Here's how the part is built. I have some questions about the finished solid (model axes, mm). A direction names the side the tool comes from. Round coordinates to 2 decimals unless told otherwise and drop trailing zeros. Loops run counter-clockwise (first coordinate to the right, second up) from the corner with the lowest first, then second, coordinate; pieces in that order, holes last. Notation, with made-up numbers: M 60,74.5 L 72,74.5 A18 cw 72,83.5 Z; hole C -6.5,-9.75 d8. An arc over 180 degrees is marked long. Write each question's results on one line, items separated by ' | '. Start each with the question number.
```python
from build123d import *

# Parameters (mm, degrees)
SKETCH2_R           = 4.75
SKETCH2_R_2         = 3.75
BOSS_EXTRUDE1_DEPTH = 3.44
SKETCH3_W           = 4
SKETCH3_H           = 11.757601451
BOSS_EXTRUDE2_DEPTH = 1
SKETCH4_W           = 1.4
SKETCH4_H           = 4.6
CUT_EXTRUDE1_DEPTH  = 1
FILLET1_R           = 13
CHAMFER1_SIZE       = 0.5
FILLET2_R           = 1


with BuildPart() as part:
    # Sketch2 → Boss-Extrude1 (new body)
    with BuildSketch(Plane(origin=(0, 0, 0), x_dir=(1, 0, 0), z_dir=(0, 1, 0))):
        with Locations(Location((0, 0, 0), (0, 0, 270))):
            Circle(SKETCH2_R)
        with Locations(Location((0, 0, 0), (0, 0, 270))):
            Circle(SKETCH2_R_2, mode=Mode.SUBTRACT)
    extrude(amount=BOSS_EXTRUDE1_DEPTH)

    # Sketch3 → Boss-Extrude2 (add)
    with BuildSketch(Plane(origin=(-4.8, 0, 0), x_dir=(0, 0, -1), z_dir=(1, 0, 0))):
        with Locations((0, 5.878800726)):
            Rectangle(SKETCH3_W, SKETCH3_H)
    extrude(amount=BOSS_EXTRUDE2_DEPTH)

    # Sketch4 → Cut-Extrude1 (cut)
    with BuildSketch(Plane.ZY.offset(4.8)):
        with Locations((0, 8.46916965)):
            Rectangle(SKETCH4_W, SKETCH4_H)
    extrude(amount=-CUT_EXTRUDE1_DEPTH, mode=Mode.SUBTRACT)

    # Fillet1
    # the kernel refuses this fillet: 13 mm, written as the material it adds along each edge
    with BuildSketch(Plane(origin=(-4.308421985, 3.44, 2), x_dir=(0.5581025465687688, 0, 0.8297719852546573), z_dir=(0, -1, 0))) as fillet1_piece_1:
        with BuildLine():
            CenterArc((3.528934631, 12.839109145), FILLET1_R, 252.988692503, 7.987692365)
            Line((-0.274350942, 0.407897665), (-0.350416654, 0.159273436))
            ThreePointArc((-0.350416654, 0.159273436), (-0.352916187, 0.058842171), (-0.215740716, -0.145106662))
            Line((-0.215740716, -0.145106662), (0.0407788, -0.256782183))
            ThreePointArc((0.0407788, -0.256782183), (0.744997311, -0.201212957), (1.449215822, -0.256782183))
            Line((1.449215822, -0.256782183), (1.489994622, 0))
        make_face()
    extrude(amount=3.44)
    with BuildSketch(Plane(origin=(-4.308421985, 3.44, -2), x_dir=(0.5581025465687675, 0, -0.8297719852546583), z_dir=(0, -1, 0))) as fillet1_piece_2:
        with BuildLine():
            CenterArc((3.528934631, -12.839109145), FILLET1_R, 99.023615132, 7.987692365)
            Line((-0.274350942, -0.407897665), (-0.350416654, -0.159273436))
            ThreePointArc((-0.350416654, -0.159273436), (-0.352916187, -0.058842171), (-0.215740716, 0.145106662))
            Line((-0.215740716, 0.145106662), (0.0407788, 0.256782183))
            ThreePointArc((0.0407788, 0.256782183), (0.744997311, 0.201212957), (1.449215822, 0.256782183))
            Line((1.449215822, 0.256782183), (1.489994622, 0))
        make_face()
    extrude(amount=3.44)

    # Chamfer1
    chamfer1_edges = [part.edges().sort_by_distance(p)[0] for p in [
        (0, 0, -3.75),
    ]]
    chamfer(chamfer1_edges, length=CHAMFER1_SIZE)

    # Fillet2
    # the kernel refuses this fillet: 1 mm, written as the material it takes off along each edge
    with BuildSketch(Plane(origin=(-4.8, 0, 4.5), x_dir=(1, 0, 0), z_dir=(0, 0, -1))) as fillet2_piece_1:
        with BuildLine():
            CenterArc((FILLET2_R, -FILLET2_R), FILLET2_R, 90, 90)
            Line((0, -FILLET2_R), (0, 0))
            Line((0, 0), (FILLET2_R, 0))
        make_face()
    extrude(amount=9, mode=Mode.SUBTRACT)
    with BuildSketch(Plane(origin=(-4.8, 11.757601451, -4.5), x_dir=(0, -1, 0), z_dir=(0, 0, 1))) as fillet2_piece_2:
        with BuildLine():
            CenterArc((FILLET2_R, FILLET2_R), FILLET2_R, 180, 90)
            Line((0, FILLET2_R), (0, 0))
            Line((0, 0), (FILLET2_R, 0))
        make_face()
    extrude(amount=9, mode=Mode.SUBTRACT)


solid = part.part
```
Item 1: I'm going to push flat-ended pins straight in: pin 1 (1.5 mm diameter, centred on y = 9.5, z = 3, fed in from +X); pin 2 (4.5 mm diameter, centred on y = 9, z = 1, fed in from +X); pin 3 (1.1 mm diameter, centred on x = -4.5, z = 0, fed in from +Y); pin 4 (0.5 mm diameter, centred on x = -4.5, y = 8, fed in from -Z). Where does each tip first touch, or does it pass through?
Item 2: If we section it at C-C on z = 0: Please give me the cut outline in (x, y), and give its area (3 significant figures).
Item 3: If we section it at D-D on y = 5.5: Please give me the cut outline in (x, z), and give its area (3 significant figures).
Item 4: If we section it at B-B on x = 0: Please give me the cut outline in (y, z).
Item 5: I need wall thicknesses on L1, parallel to X at y = 8, z = 0.75; L2, parallel to Z at x = 3, y = 3.25; L3, parallel to Z at x = 2.5, y = 1.5. Which ranges of each line are inside material? Lowest first, please.
Item 6: Which directions (+Z, -Z, +X, -X, +Y, -Y) give clear straight access to the entire face, cutting with the end or side of a thin tool? Please do faces 4 (the face through (-4, 8, 0.7)), 5 (the face through (-4, 8, 2)), 6 (the face through (-4, 8, -2)), 7 (the face through (-4.8, 6, 0)), 8 (the face through (-3.8, 8, 1)).
Item 7: If we section it at A-A on y = 8.25: Please give me the cut outline in (x, z), and give its area (3 significant figures).
Item 8: If we mould it in two halves opening along X, with no side actions, what happens to faces 1 (the face through (-4, 6.169, 0)), 2 (the face through (-4.126, 1.744, 2.586)), 3 (the face through (0.165, 1.949, -3.746))? For each: released by +X, released by -X, zero draft, split by the parting line, or undercut.
Numbers:
1) pin 1: through | pin 2: x = -3.8 | pin 3: y = 11.75 | pin 4: z = -2
2) outline: M -4.8,1 A1 ccw -4.18,0.07 L -3.75,0.5 L -3.75,3.44 L -3.8,3.44 L -3.8,6.17 L -4.8,6.17 Z; M -4.8,10.77 L -3.8,10.77 L -3.8,11.76 A1 ccw Z; M 3.75,0.5 L 4.25,0 L 4.75,0 L 4.75,3.44 L 3.75,3.44 Z | area: 10.1 mm²
3) outline: M -4.8,-2 L -3.8,-2 L -3.8,2 L -4.8,2 Z | area: 4.00 mm²
4) outline: M 0,-4.75 L 3.44,-4.75 L 3.44,-3.75 L 0.5,-3.75 L 0,-4.25 Z; M 0,4.25 L 0.5,3.75 L 3.44,3.75 L 3.44,4.75 L 0,4.75 Z
5) L1: -4.8 to -3.8 | L2: -3.68 to -2.25, 2.25 to 3.68 | L3: -4.04 to -2.8, 2.8 to 4.04
6) face 4: +X, -X | face 5: +Z, +X, -X, +Y | face 6: -Z, +X, -X, +Y | face 7: +Z, -Z, -X, +Y, -Y | face 8: +Z, -Z, +X, +Y
7) outline: M -4.8,-2 L -3.8,-2 L -3.8,-0.7 L -4.8,-0.7 Z; M -4.8,0.7 L -3.8,0.7 L -3.8,2 L -4.8,2 Z | area: 2.60 mm²
8) face 1: zero draft | face 2: released by -X | face 3: undercut
